Autodesk Inventor part; units mm, degrees
ref_plane "Work Plane1" through (0, 304.8, 0) normal (0, 1, 0) x (1, 0, 0)
ref_plane "YZ Plane" through (0, 0, 0) normal (1, 0, 0) x (0, 1, 0)
ref_plane "XZ Plane" through (0, 0, 0) normal (0, 1, 0) x (-1, 0, 0)
sketch "Sketch1" plane through (0, 0, 0) normal (0, 0, 1) x (1, 0, 0)
  line L0 (0, 0) -> (254, 0)
  line L1 (254, 0) -> (254, 355.6)
  line L2 (254, 355.6) -> (0, 355.6)
  line L3 (0, 355.6) -> (0, 0)
  dimension "d0" = 254
  dimension "d1" = 355.6
extrude "Extrusion1" add sketch "Sketch1" along normal blind 6.35
sketch "Sketch2" plane through (0, 0, 6.35) normal (0, 0, 1) x (1, 0, 0)
  line L0 (38.1, 342.9) -> (215.9, 342.9) construction
  line L1 (241.3, 317.5) -> (241.3, 38.1) construction
  line L2 (215.9, 12.7) -> (38.1, 12.7) construction
  line L3 (12.7, 38.1) -> (12.7, 317.5) construction
  line L4 (0, 355.6) -> (0, 0) construction
  line L5 (254, 355.6) -> (0, 355.6) construction
  arc A0 (241.3, 317.5) -> (215.9, 342.9) centre (215.9, 317.5) ccw construction
  arc A1 (38.1, 342.9) -> (12.7, 317.5) centre (38.1, 317.5) ccw construction
  arc A2 (12.7, 38.1) -> (38.1, 12.7) centre (38.1, 38.1) ccw construction
  arc A3 (215.9, 12.7) -> (241.3, 38.1) centre (215.9, 38.1) ccw construction
  line L6 (215.9, 38.1) -> (233.8605, 20.1395) construction
  line L7 (38.1, 38.1) -> (20.1395, 20.1395) construction
  line L8 (38.1, 317.5) -> (20.1395, 335.4605) construction
  line L9 (215.9, 317.5) -> (233.8605, 335.4605) construction
  circle A4 centre (20.1395, 335.4605) radius 3.1
  circle A5 centre (233.8605, 335.4605) radius 3.1
  circle A6 centre (233.8605, 20.1395) radius 3.1
  circle A7 centre (20.1395, 20.1395) radius 3.1
  circle A8 centre (12.7, 38.1) radius 3.1
  circle A9 centre (38.1, 12.7) radius 3.1
  circle A10 centre (215.9, 12.7) radius 3.1
  circle A11 centre (241.3, 38.1) radius 3.1
  circle A12 centre (241.3, 317.5) radius 3.1
  circle A13 centre (215.9, 342.9) radius 3.1
  circle A14 centre (38.1, 342.9) radius 3.1
  circle A15 centre (12.7, 317.5) radius 3.1
  circle A16 centre (241.3, 282.575) radius 3.1
  circle A17 centre (241.3, 247.65) radius 3.1
  circle A18 centre (241.3, 212.725) radius 3.1
  circle A19 centre (241.3, 177.8) radius 3.1
  circle A20 centre (241.3, 142.875) radius 3.1
  circle A21 centre (180.34, 342.9) radius 3.1
  circle A22 centre (144.78, 342.9) radius 3.1
  circle A23 centre (109.22, 342.9) radius 3.1
  circle A24 centre (73.66, 342.9) radius 3.1
  circle A25 centre (180.34, 12.7) radius 3.1
  circle A26 centre (144.78, 12.7) radius 3.1
  circle A27 centre (109.22, 12.7) radius 3.1
  circle A28 centre (73.66, 12.7) radius 3.1
  circle A29 centre (241.3, 107.95) radius 3.1
  circle A30 centre (241.3, 73.025) radius 3.1
  circle A31 centre (241.3, 38.1) radius 3.1
  circle A32 centre (12.7, 282.575) radius 3.1
  circle A33 centre (12.7, 247.65) radius 3.1
  circle A34 centre (12.7, 212.725) radius 3.1
  circle A35 centre (12.7, 177.8) radius 3.1
  circle A36 centre (12.7, 142.875) radius 3.1
  circle A37 centre (12.7, 107.95) radius 3.1
  circle A38 centre (12.7, 73.025) radius 3.1
  point P0 (241.3, 12.7)
  point P1 (241.3, 342.9)
  point P2 (12.7, 12.7)
  dimension "d4" = 228.6
  dimension "d5" = 330.2
  dimension "d6" = 12.7
  dimension "d7" = 12.7
  dimension "d8" = 25.4
  dimension "d9" = 6.2
  dimension "d10" = 6.2
  dimension "d11" = 6.2
  dimension "d12" = 6.2
  dimension "d13" = 6.2
  dimension "d14" = 6.2
  dimension "d15" = 6.2
  dimension "d16" = 6.2
  dimension "d17" = 6.2
  dimension "d18" = 6.2
  dimension "d19" = 6.2
  dimension "d20" = 6.2
  dimension "d30" = 34.925
  dimension "d37" = 35.56
  dimension "d44" = 35.56
  dimension "d51" = 0
  dimension "d52" = 0
  dimension "d53" = 0
  dimension "d54" = 0
  dimension "d57" = 34.925
extrude "Extrusion2" cut sketch "Sketch2" against normal blind 12.7
sketch "Sketch3" plane through (0, 0, 6.35) normal (0, 0, 1) x (1, 0, 0)
  line L0 (38.1, 335.28) -> (215.9, 335.28)
  line L1 (233.68, 317.5) -> (233.68, 38.1)
  line L2 (215.9, 20.32) -> (38.1, 20.32)
  line L3 (20.32, 38.1) -> (20.32, 317.5)
  line L4 (254, 355.6) -> (0, 355.6)
  line L5 (0, 355.6) -> (0, 0)
  arc A0 (38.1, 335.28) -> (20.32, 317.5) centre (38.1, 317.5) ccw
  arc A1 (233.68, 317.5) -> (215.9, 335.28) centre (215.9, 317.5) ccw
  arc A2 (215.9, 20.32) -> (233.68, 38.1) centre (215.9, 38.1) ccw
  arc A3 (20.32, 38.1) -> (38.1, 20.32) centre (38.1, 38.1) ccw
  point P0 (233.68, 20.32)
  point P1 (233.68, 335.28)
  point P2 (20.32, 20.32)
  dimension "d62" = 213.36
  dimension "d63" = 314.96
  dimension "d64" = 20.32
  dimension "d65" = 20.32
  dimension "d66" = 17.78
ref_plane "Work Plane1" through (0, 304.8, 0) normal (0, 1, 0) x (1, 0, 0)
sketch "Sketch5" plane through (0, 304.8, 0) normal (0, 1, 0) x (1, 0, 0)
  line L0 (0, -6.35) -> (254, -6.35)
  circle A0 centre (20.32, -6.35) radius 3.175
  line L1 (0, 0) -> (0, -6.35)
  dimension "d70" = 6.35
  dimension "d71" = 20.32
sweep "Sweep1" cut profiles "Sketch5" path "Sketch3" path curves L3 A3 L2 A2 L1 A1 L0 A0
sketch "Sketch6" plane through (0, 0, 6.35) normal (0, 0, 1) x (1, 0, 0)
  line L0 (38.1, 330.2) -> (215.9, 330.2)
  line L1 (228.6, 317.5) -> (228.6, 38.1)
  line L2 (215.9, 25.4) -> (38.1, 25.4)
  line L3 (25.4, 38.1) -> (25.4, 317.5)
  line L4 (0, 355.6) -> (0, 0)
  line L5 (254, 355.6) -> (0, 355.6)
  arc A0 (38.1, 330.2) -> (25.4, 317.5) centre (38.1, 317.5) ccw
  arc A1 (228.6, 317.5) -> (215.9, 330.2) centre (215.9, 317.5) ccw
  arc A2 (215.9, 25.4) -> (228.6, 38.1) centre (215.9, 38.1) ccw
  arc A3 (25.4, 38.1) -> (38.1, 25.4) centre (38.1, 38.1) ccw
  point P0 (228.6, 25.4)
  point P1 (228.6, 330.2)
  point P2 (25.4, 25.4)
  dimension "d74" = 203.2
  dimension "d75" = 304.8
  dimension "d76" = 25.4
  dimension "d77" = 25.4
  dimension "d78" = 12.7
extrude "Extrusion3" cut sketch "Sketch6" against normal blind 25.4
properties part number "alumbottom3" material "Aluminum 6061"
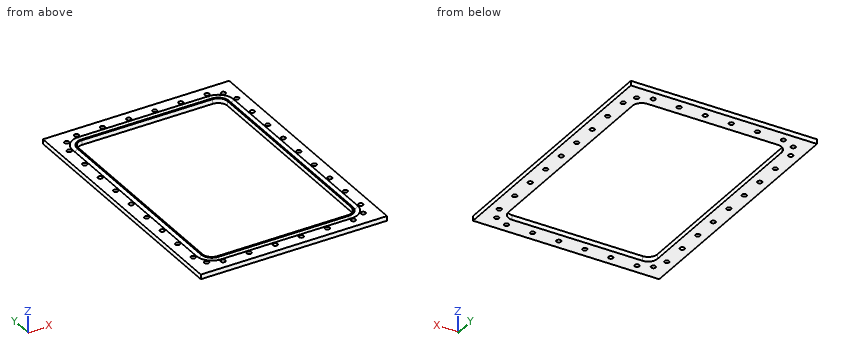
Input: part model. Units: mm. Frame: model coordinates. Coordinates: 2 decimals unless noted, no trailing zeros. Loops run counter-clockwise (first coordinate to the right, second up) from the corner with the lowest first, then second, coordinate; pieces in that order, holes last. Notation, with made-up numbers: M 30.25,66 L 52.25,66 A11 cw 52.25,71 Z; hole C 55,49 d9. An arc over 180 degrees is marked long. One line per item, written item: value.
(1) Section A-A (x = 64). Output: boundary loops of the cut face in (y, z) (3 decimals), and give its area (3 significant figures).
Filled in:
outline: M 0,0 L 25.4,0 L 25.4,6.35 L 23.495,6.35 A3.175 cw 17.145,6.35 L 0,6.35 Z; M 330.2,0 L 355.6,0 L 355.6,6.35 L 338.455,6.35 A3.175 cw 332.105,6.35 L 330.2,6.35 Z
area: 291 mm^2
(2) Section B-B (y = 308). Output: boundary loops of the cut face in (x, z) (3 decimals).
Filled in:
outline: M 0,0 L 25.4,0 L 25.4,6.35 L 23.495,6.35 A3.175 cw 17.145,6.35 L 0,6.35 Z; M 228.6,0 L 254,0 L 254,6.35 L 236.855,6.35 A3.175 cw 230.505,6.35 L 228.6,6.35 Z
(3) Line query: line 1 along Y through (x, z) = (73.66, 1.5); line 2 along Y through (x, z) = (106.5, 4.5); line 3 along X through (y, z) = (157, 4). Output: solid intervals per line, ascending. Write a range as from..to.
Filled in:
line 1: 0..9.6, 15.8..25.4, 330.2..339.8, 346..355.6
line 2: 0..11.21, 14.19..17.74, 22.9..25.4, 330.2..332.7, 337.86..341.41, 344.39..355.6
line 3: 0..18.19, 22.45..25.4, 228.6..231.55, 235.81..254
(4) Section C-C (z = 4.75). Give the number of separate pieces and of enclosed holes in the cut face, and give its area (3 significant figures).
Filled in:
separate pieces: 2
enclosed holes: 36
area: 21,900 mm^2
